Can you work these out from the drawing? Everything is in mm from the part's minimum corner. Coordinates: 2 decimals unless noted, no trailing zeros. Loops run counter-clockwise (first coordinate to the right, second up) from the corner with the lowest first, then second, coordinate; pieces in that order, holes last. Notation, with made-up numbers: (-5.5, 17) - (16.5, 17) arc R36 ccw to (16.5, 52) - close; hole circle Ø3 at (-1, 75). An arc over 180 degrees is marked (long way). Use CSV: the item, a comma, the result in double quotes.
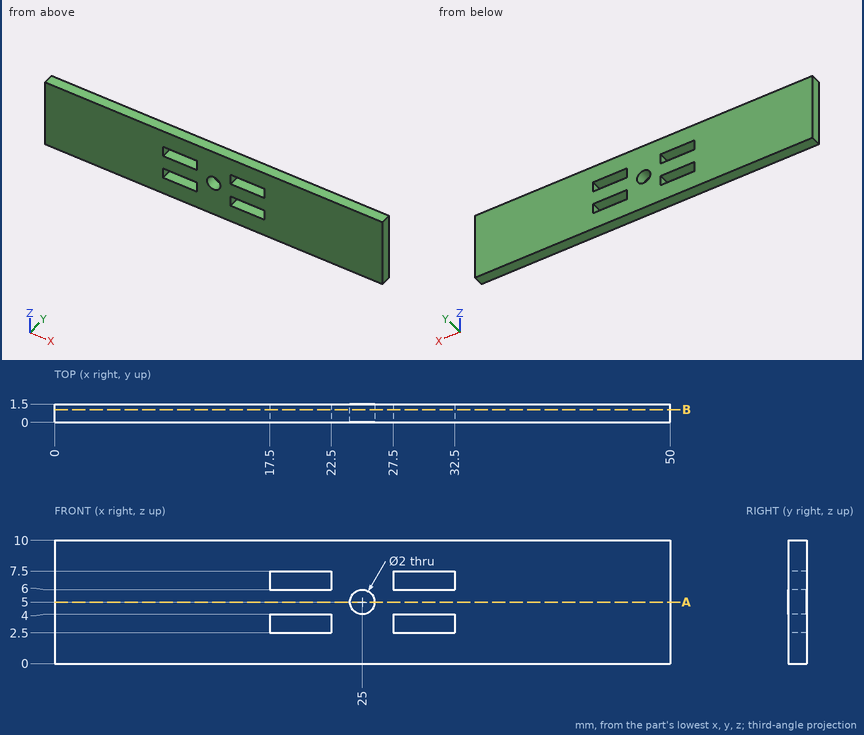
(1) Please list where these lines run through material, in increasing order: line 1 (X direction, y = 0.6, z = 3.5); line 2 (Z direction, x = 25, y = 1.2); line 3 (Z direction, x = 28, y = 1.3).
Computed:
line 1,"x = 0 to 17.5, 22.5 to 27.5, 32.5 to 50"
line 2,"z = 0 to 4, 6 to 10"
line 3,"z = 0 to 2.5, 4 to 6, 7.5 to 10"
(2) Suppose I cut it at A-A (z = 5). Write out the boundary of the cut face in (x, y), plus the area to 3 significant figures.
Computed:
outline,"(0, 0) - (24, 0) - (24, 1.5) - (0, 1.5) - close; (26, 0) - (50, 0) - (50, 1.5) - (26, 1.5) - close"
area,"72.0 mm²"
(3) Suppose I cut it at B-B (y = 1.05). Write out the boundary of the cut face in (x, z), plus the area to 3 significant figures.
Computed:
outline,"(0, 0) - (50, 0) - (50, 10) - (0, 10) - close; hole (17.5, 2.5) - (22.5, 2.5) - (22.5, 4) - (17.5, 4) - close; hole (17.5, 6) - (22.5, 6) - (22.5, 7.5) - (17.5, 7.5) - close; hole circle Ø2 at (25, 5); hole (27.5, 2.5) - (32.5, 2.5) - (32.5, 4) - (27.5, 4) - close; hole (27.5, 6) - (32.5, 6) - (32.5, 7.5) - (27.5, 7.5) - close"
area,"467 mm²"
